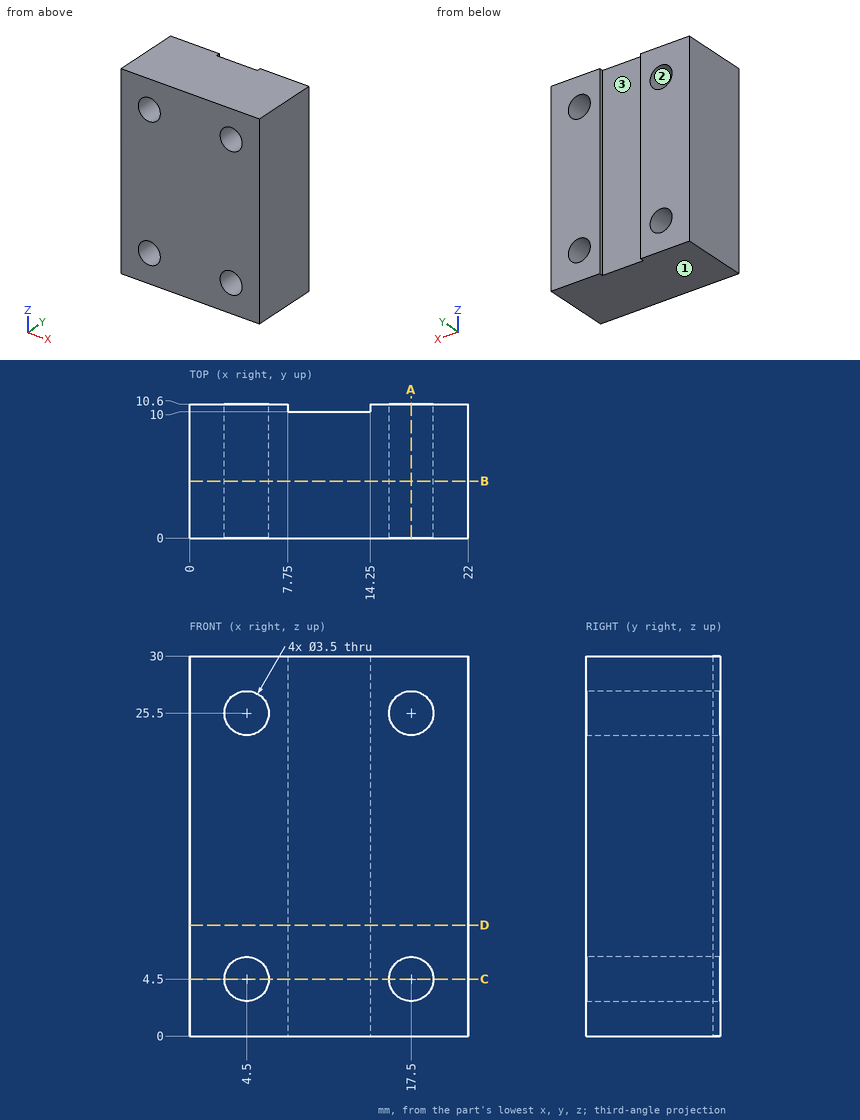
Job drawing, mm, ordinate dimensions from the low corner. One solid piece. Give positions to 0.01 mm unless a question says otherwise; leave off trailing zeros. Order: outer loops, then holes, each group sorted by start corner. A loop starts at its lowest first (then second) coordinate and runs counter-clockwise, first axis right, second up. Notation, with made-up numbers: M 25.25,-16 L 49.25,-16 A37 ccw 49.25,23 Z; hole C -33,-3.75 d3. An arc over 180 degrees is marked long. Put each result on its own line as item: value. Start each with the question number.
(1) Pull direction Z, two halves, no side cores. Call the marked faces 1, 2 and 3: released by +Z, released by -Z, zero draft, split by the parting line, or undercut.
(2) Band-saw the part on D-D on z = 8.75. Give the cut face in (x, y), then the cut area to 3 significant figures.
(3) Drill centre lines: L1, parallel to X at y = 4, z = 25.5; L2, parallel to Y at x = 12.25, z = 11.5. Where is each one in solid material? Low to high. Write a range as [from, to].
(4) Pin check, flat tip, straight feed: pin 1 Ø5 at (x, z) = (11.5, 14.5) entering from +Y. Stop position of the tip, or through.
(5) Band-saw the part on B-B on y = 4.5. Give the cut face in (x, z), then the cut area to 3 significant figures.
(6) Band-saw the part on C-C on z = 4.5. Give the cut face in (x, y).
(7) Band-saw the part on A-A on x = 17.5. Give the cut face in (y, z).
Results below:
1. face 1: released by -Z
1. face 2: undercut
1. face 3: zero draft
2. outline: M 0,0 L 22,0 L 22,10.6 L 14.25,10.6 L 14.25,10 L 7.75,10 L 7.75,10.6 L 0,10.6 Z
2. area: 229 mm2
3. L1: x = [0, 2.75], [6.25, 15.75], [19.25, 22]
3. L2: y = [0, 10]
4. pin 1: stops at y = 10
5. outline: M 0,0 L 22,0 L 22,30 L 0,30 Z; hole C 4.5,4.5 d3.5; hole C 4.5,25.5 d3.5; hole C 17.5,4.5 d3.5; hole C 17.5,25.5 d3.5
5. area: 622 mm2
6. outline: M 0,0 L 2.75,0 L 2.75,10.6 L 0,10.6 Z; M 6.25,0 L 15.75,0 L 15.75,10.6 L 14.25,10.6 L 14.25,10 L 7.75,10 L 7.75,10.6 L 6.25,10.6 Z; M 19.25,0 L 22,0 L 22,10.6 L 19.25,10.6 Z
7. outline: M 0,0 L 10.6,0 L 10.6,2.75 L 0,2.75 Z; M 0,6.25 L 10.6,6.25 L 10.6,23.75 L 0,23.75 Z; M 0,27.25 L 10.6,27.25 L 10.6,30 L 0,30 Z
